Geometry: final body of the model. Coordinates: model frame, mm. A direction names the side the tool comes from. Coordinates: 2 decimals unless noted, no trailing zeros. Order: outer loops, then holes, each group sorted by start corner. A loop starts at its lowest first (then second) coordinate and runs counter-clockwise, first axis right, second up. Notation, with made-up numbers: M -14,47 L 35,47 A29 cw 35,79 Z; hole C 85,63 d1. An arc over 180 degrees is marked long. Use CSV: the item, a comma, the result in double quotes. Start each with the question number.
1. Pull-direction query (X, two-part tool) for faces 1 (the cylindrical face through (0.66, -60.038, 39.985)), 2 (the flat face through (0, 22.5, 25)), 3 (the cylindrical face through (-14.07, 15.95, 1.97)), 4 (the flat face through (22.5, 0, 24)); classes: pulls with the +X half, pulls with the -X half, needs draft (parallel to the pull), parting line crosses it, or undercut.
2. Section query C-C on x = 0. Return the cut outline in (y, z).
3. First-contact query: P1, Ø0.7, axis at x = 22, z = 47.5, coming from the +Y side; P2, Ø5, axis at y = -42, z = 40.5, coming from the -X side; P3, Ø2.5, axis at x = 15.5, y = -15.5, coming from the -Z side; P4, Ø5, axis at x = -15.5, y = -15.5, coming from the +Z side. Flat tips, straight axial feed; report the tip coordinate or a pass-through.
4. Section query B-B on z = 25. Return the cut outline in (x, y).
5. Section query D-D on y = -12. Return the cut outline in (x, z).
6. Section query A-A on y = 0. Return the cut outline in (x, z), and give its area (3 significant figures).
7. Set-up query: faces 5 (the cylindrical face through (16.93, 15.95, 1.97)), 6 (the flat face through (-19, -22.5, 14)), 7 (the cylindrical face through (20.25, 20.29, 26.68)). Return all of +Z, -Z, +X, -X, +Y, -Y with unobstructed straight access to the full face (end or side cutting, diameter ignored); none if empty.
8. Material intervals for line 1 (Y direction, x = 9, z = 6); line 2 (X direction, y = 0, z = 2), sorted ascending.
from build123d import *

# Parameters (mm, degrees)
SKETCH1_W               = 45
SKETCH1_H               = 45
BOSS_EXTRUDE1_DEPTH     = 50
SKETCH2_W               = 42.3
SKETCH2_H               = 42.3
CUT_EXTRUDE1_DEPTH      = 46
CUT_EXTRUDE2_DEPTH      = 56.932995629
CUT_EXTRUDE2_DEPTH_BACK = 56.932995629
SKETCH3_R               = 1.5
SKETCH3_R_2             = 2.75
SKETCH4_R               = 15
BOSS_EXTRUDE2_DEPTH     = 71
FILLET1_R               = 2
FILLET2_R               = 5
FILLET3_R               = 3
SKETCH7_W               = 5
SKETCH7_H               = 10
CUT_EXTRUDE3_DEPTH      = 10


with BuildPart() as part:
    # Sketch1 → Boss-Extrude1 (new body)
    with BuildSketch(Plane.XY):
        Rectangle(SKETCH1_W, SKETCH1_H)
    extrude(amount=BOSS_EXTRUDE1_DEPTH)

    # Sketch2 → Cut-Extrude1 (cut)
    with BuildSketch(Plane.XY.offset(50)):
        Rectangle(SKETCH2_W, SKETCH2_H)
    extrude(amount=-CUT_EXTRUDE1_DEPTH, mode=Mode.SUBTRACT)

    # Sketch3 → Cut-Extrude2 (cut, two sides: drawn at the far end of the back side and taken through both)
    with BuildSketch(Plane.XY.offset(4).offset(-CUT_EXTRUDE2_DEPTH_BACK)):
        with Locations((-15.499780644, 15.499780644)):
            Circle(SKETCH3_R)
        with Locations((15.499780644, 15.499780644)):
            Circle(SKETCH3_R)
        with Locations((15.499780644, -15.499780644)):
            Circle(SKETCH3_R)
        with Locations((-15.499780644, -15.499780644)):
            Circle(SKETCH3_R)
        Circle(SKETCH3_R_2)
    extrude(amount=CUT_EXTRUDE2_DEPTH + CUT_EXTRUDE2_DEPTH_BACK, mode=Mode.SUBTRACT)

    # Sketch4 → Boss-Extrude2 (add)
    with BuildSketch(Plane.XZ.offset(22.5)):
        with Locations(Location((0, 25, 0), (0, 0, 270))):
            Circle(SKETCH4_R)
    extrude(amount=BOSS_EXTRUDE2_DEPTH)

    # Fillet1
    # the kernel refuses this fillet: 2 mm, written as the material it takes off along each edge
    with BuildSketch(Plane(origin=(-22.5, -27.5, 50), x_dir=(0, 0, -1), z_dir=(0, 1, 0)), Plane(origin=(22.5, 27.5, 50), x_dir=(0, 0, -1), z_dir=(0, -1, 0))) as fillet1_piece_1:
        with BuildLine():
            CenterArc((FILLET1_R, -FILLET1_R), FILLET1_R, 90, 90)
            Line((0, -FILLET1_R), (0, 0))
            Line((0, 0), (FILLET1_R, 0))
        make_face()
    extrude(amount=55, mode=Mode.SUBTRACT)
    with BuildSketch(Plane(origin=(22.5, -22.5, -5), x_dir=(0, 1, 0), z_dir=(0, 0, 1)), Plane(origin=(22.5, 22.5, -5), x_dir=(-1, 0, 0), z_dir=(0, 0, 1))) as fillet1_piece_2:
        with BuildLine():
            CenterArc((FILLET1_R, FILLET1_R), FILLET1_R, 180, 90)
            Line((0, FILLET1_R), (0, 0))
            Line((0, 0), (FILLET1_R, 0))
        make_face()
    extrude(amount=60, mode=Mode.SUBTRACT)
    with BuildSketch(Plane(origin=(-22.5, -22.5, -5), x_dir=(0, 1, 0), z_dir=(0, 0, 1)), Plane(origin=(-22.5, 22.5, -5), x_dir=(1, 0, 0), z_dir=(0, 0, 1))) as fillet1_piece_3:
        with BuildLine():
            CenterArc((FILLET1_R, -FILLET1_R), FILLET1_R, 90, 90)
            Line((0, -FILLET1_R), (0, 0))
            Line((0, 0), (FILLET1_R, 0))
        make_face()
    extrude(amount=60, mode=Mode.SUBTRACT)

    # Fillet2
    fillet2_edges = [part.edges().sort_by_distance(p)[0] for p in [
        (0, -22.5, 40),
    ]]
    fillet(fillet2_edges, radius=FILLET2_R)

    # Fillet3
    fillet3_edges = [part.edges().sort_by_distance(p)[0] for p in [
        (-21.15, -21.15, 26.945714016),
        (21.15, 21.15, 26.945714016),
        (-21.15, 21.15, 26.945714016),
        (21.15, -21.15, 26.945714016),
    ]]
    fillet(fillet3_edges, radius=FILLET3_R)

    # Sketch7 → Cut-Extrude3 (cut)
    with BuildSketch(Plane(origin=(22.5, 0, 0), x_dir=(0, 0, -1), z_dir=(1, 0, 0))):
        with Locations((-47.391428032, 0)):
            Rectangle(SKETCH7_W, SKETCH7_H)
    extrude(amount=-CUT_EXTRUDE3_DEPTH, mode=Mode.SUBTRACT)


solid = part.part
Results list:
1,face 1,"parting line crosses it"
1,face 2,"needs draft"
1,face 3,"undercut"
1,face 4,"pulls with the +X half"
2,outline,"M -93.5,10 L -27.5,10 A5 cw -22.5,5 L -22.5,0 L -2.75,0 L -2.75,4 L -21.15,4 L -21.15,50 L -22.5,50 L -22.5,45 A5 cw -27.5,40 L -93.5,40 Z; M 2.75,0 L 22.5,0 L 22.5,50 L 21.15,50 L 21.15,4 L 2.75,4 Z"
3,P1,"stops at y = 22.14"
3,P2,"stops at x = -7.48"
3,P3,"passes through"
3,P4,"stops at z = 4"
4,outline,"M -22.5,-20.5 A2 ccw -20.5,-22.5 L -20,-22.5 A5 cw -15,-27.5 L -15,-93.5 L 15,-93.5 L 15,-27.5 A5 cw 20,-22.5 L 20.5,-22.5 A2 ccw 22.5,-20.5 L 22.5,20.5 A2 ccw 20.5,22.5 L -20.5,22.5 A2 ccw -22.5,20.5 Z; hole M -21.15,-18.15 A3 ccw -18.15,-21.15 L 18.15,-21.15 A3 ccw 21.15,-18.15 L 21.15,18.15 A3 ccw 18.15,21.15 L -18.15,21.15 A3 ccw -21.15,18.15 Z"
5,outline,"M -22.5,0 L 22.5,0 L 22.5,48 A2 ccw 21.15,49.89 L 21.15,4 L -21.15,4 L -21.15,49.89 A2 ccw -22.5,48 Z"
6,outline,"M -22.5,0 L -2.75,0 L -2.75,4 L -21.15,4 L -21.15,49.89 A2 ccw -22.5,48 Z; M 2.75,0 L 22.5,0 L 22.5,44.89 L 21.15,44.89 L 21.15,4 L 2.75,4 Z"
6,area,"274 mm²"
7,face 5,"+Z, -Z"
7,face 6,"-Y"
7,face 7,"+Z"
8,line 1,"y = -22.5 to -21.15, 21.15 to 22.5"
8,line 2,"x = -22.5 to -2.75, 2.75 to 22.5"
